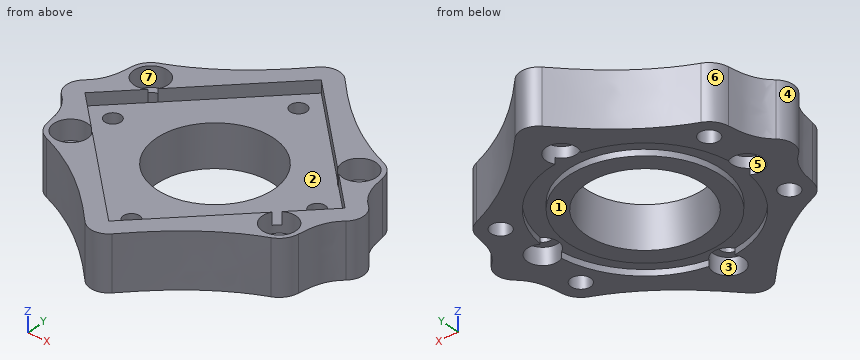
```python
from build123d import *

# Parameters (mm, degrees)
MAIN_FEATURES_SKETCH_R         = 19.05
MAIN_BODY_DEPTH                = 17.78
SKETCH1_8_R                    = 31
SKETCH1_8_R_2                  = 25
RING_POCKET_DEPTH              = 2
CBORE_FOR_M6_SHCS1_D           = 6.4
CBORE_FOR_M6_SHCS1_CBORE_D     = 11
CBORE_FOR_M6_SHCS1_CBORE_DEPTH = 6.5
CBORE_FOR_M5_SHCS1_D           = 5.3
CBORE_FOR_M5_SHCS1_CBORE_D     = 10
CBORE_FOR_M5_SHCS1_CBORE_DEPTH = 5.5
CUT_EXTRUDE5_START             = 17.78
CUT_EXTRUDE5_DEPTH             = 4


with BuildPart() as part:
    # main_features_sketch → main_body (new body)
    with BuildSketch(Plane.XY):
        with BuildLine():
            add(Edge.make_bspline(
                [(4.384277331, -46.522516279), (11.494410565, -38.912173671), (21.620981626, -28.654243233), (36.660389066, -22.474745556)],
                knots=[0, 0, 0, 0, 1, 1, 1, 1], degree=3))
            ThreePointArc((36.660389066, -22.474745556), (39.572504615, -20.236412671), (40.950412855, -16.831721795))
            add(Edge.make_bspline(
                [(40.950412855, -16.831721795), (41.488925466, -12.331557199), (42.397215407, -7.970955774), (46.359831988, -4.530802009)],
                knots=[0, 0, 0, 0, 1, 1, 1, 1], degree=3))
            ThreePointArc((46.359831988, -4.530802009), (48.426406871, 0), (46.359831988, 4.530802009))
            add(Edge.make_bspline(
                [(40.950412855, 16.831721795), (41.488925466, 12.331557199), (42.397215407, 7.970955774), (46.359831988, 4.530802009)],
                knots=[0, 0, 0, 0, 1, 1, 1, 1], degree=3))
            ThreePointArc((40.950412855, 16.831721795), (39.572504615, 20.236412671), (36.660389066, 22.474745556))
            add(Edge.make_bspline(
                [(4.384277331, 46.522516279), (11.494410565, 38.912173671), (21.620981626, 28.654243233), (36.660389066, 22.474745556)],
                knots=[0, 0, 0, 0, 1, 1, 1, 1], degree=3))
            ThreePointArc((4.384277331, 46.522516279), (0, 48.426406871), (-4.384277331, 46.522516279))
            add(Edge.make_bspline(
                [(-4.384277331, 46.522516279), (-11.494410565, 38.912173671), (-21.620981626, 28.654243233), (-36.660389066, 22.474745556)],
                knots=[0, 0, 0, 0, 1, 1, 1, 1], degree=3))
            ThreePointArc((-36.660389066, 22.474745556), (-39.572504615, 20.236412671), (-40.950412855, 16.831721795))
            add(Edge.make_bspline(
                [(-40.950412855, 16.831721795), (-41.488925466, 12.331557199), (-42.397215407, 7.970955774), (-46.359831988, 4.530802009)],
                knots=[0, 0, 0, 0, 1, 1, 1, 1], degree=3))
            ThreePointArc((-46.359831988, 4.530802009), (-48.426406871, 0), (-46.359831988, -4.530802009))
            add(Edge.make_bspline(
                [(-40.950412855, -16.831721795), (-41.488925466, -12.331557199), (-42.397215407, -7.970955774), (-46.359831988, -4.530802009)],
                knots=[0, 0, 0, 0, 1, 1, 1, 1], degree=3))
            ThreePointArc((-40.950412855, -16.831721795), (-39.572504615, -20.236412671), (-36.660389066, -22.474745556))
            add(Edge.make_bspline(
                [(-4.384277331, -46.522516279), (-11.494410565, -38.912173671), (-21.620981626, -28.654243233), (-36.660389066, -22.474745556)],
                knots=[0, 0, 0, 0, 1, 1, 1, 1], degree=3))
            ThreePointArc((-4.384277331, -46.522516279), (0, -48.426406871), (4.384277331, -46.522516279))
        make_face()
        with Locations(Location((0, 0, 0), (0, 0, 180))):
            Circle(MAIN_FEATURES_SKETCH_R, mode=Mode.SUBTRACT)
    extrude(amount=MAIN_BODY_DEPTH)

    # Sketch1<8> → ring_pocket (cut)
    with BuildSketch(Plane.XY):
        Circle(SKETCH1_8_R)
        Circle(SKETCH1_8_R_2, mode=Mode.SUBTRACT)
    extrude(amount=RING_POCKET_DEPTH, mode=Mode.SUBTRACT)

    # CBORE for M6 SHCS1 (through all)
    with Locations(Plane.XY.offset(17.78)):
        with Locations((-34, 16), (-34, -16), (34, -16), (34, 16)):
            CounterBoreHole(CBORE_FOR_M6_SHCS1_D / 2, CBORE_FOR_M6_SHCS1_CBORE_D / 2, CBORE_FOR_M6_SHCS1_CBORE_DEPTH)

    # CBORE for M5 SHCS1 (through all)
    with Locations(Plane(origin=(0, 0, 0), x_dir=(-1, 0, 0), z_dir=(0, 0, -1))):
        with Locations((0, 33.335), (33.335, 0), (0, -33.335), (-33.335, 0)):
            CounterBoreHole(CBORE_FOR_M5_SHCS1_D / 2, CBORE_FOR_M5_SHCS1_CBORE_D / 2, CBORE_FOR_M5_SHCS1_CBORE_DEPTH)

    # main_features_sketch<9> → Cut-Extrude5 (cut)
    with BuildSketch(Plane.XY.offset(CUT_EXTRUDE5_START)):
        Polygon((0, 42.426406871), (42.426406871, 0), (0, -42.426406871), (-42.426406871, 0), align=None)
    extrude(amount=-CUT_EXTRUDE5_DEPTH, mode=Mode.SUBTRACT)


solid = part.part
```
Verification items for the finished model (mm, model axes). Face numbers are marked on the shaded views. A direction names the side the tool comes from. Give positions to 0.01 mm unless a question says otherwise; leave off trailing zeros. Answer as CSV lines item,"result". Start each with the question number.
Item 1: Gauge pin test, flat ends, axial feed: pin 1 (8 mm diameter, centred on x = 0, y = 33.335, fed in from +Z); pin 2 (10 mm diameter, centred on x = 19, z = 3, fed in from +Y); pin 3 (6 mm diameter, centred on x = 0, y = 33.335, fed in from -Z); pin 4 (6 mm diameter, centred on x = -34, y = 16, fed in from -Z). Record the tip position at first contact, or that the pin passes through.
Item 2: Mould release check, pull along X, two halves, no side actions. Record for the marked faces 1, 2, 3 and 4: released by +X, released by -X, zero draft, split by the parting line, or undercut.
Item 3: Section check A-A, the plane x = 34. State how many separate pieces and enclosed holes the cut face has, plus the area to 3 significant figures.
Item 4: Access from +Z, -Z, +X, -X, +Y, -Y to the whole of each face (thin tool, end or side, straight path). Record for the marked faces 5, 6 and 7.
Item 5: Material ranges on L1, parallel to Y at x = 0, z = 10.5 (3 decimals); L2, parallel to X at y = -15, z = 3; L3, parallel to Y at x = -32.5, z = 16.5, recorded low to high.
Filled in:
1,pin 1,"z = 13.78"
1,pin 2,"y = 36.98"
1,pin 3,"z = 5.5"
1,pin 4,"through"
2,face 1,"zero draft"
2,face 2,"undercut"
2,face 3,"undercut"
2,face 4,"released by -X"
3,separate pieces,"4"
3,enclosed holes,"0"
3,area,"389 mm^2"
4,face 5,"-Z"
4,face 6,"+Z, -Z, -X, +Y"
4,face 7,"+Z"
5,L1,"-48.426 to -35.985, -30.685 to -19.05, 19.05 to 30.685, 35.985 to 48.426"
5,L2,"-41.2 to -37.04, -30.96 to -11.74, 11.74 to 30.96, 37.04 to 41.2"
5,L3,"-24.34 to -21.29, -10.71 to -9.93, 9.93 to 10.71, 21.29 to 24.34"
